Source: three-view drawing plus pictorial views. Frame: mm from the lowest corner of the part. A direction names the side the tool comes from. Give positions to 0.01 mm unless a question says otherwise; leave off trailing zeros. Loops run counter-clockwise (first coordinate to the right, second up) from the corner with the lowest first, then second, coordinate; pieces in that order, holes last.
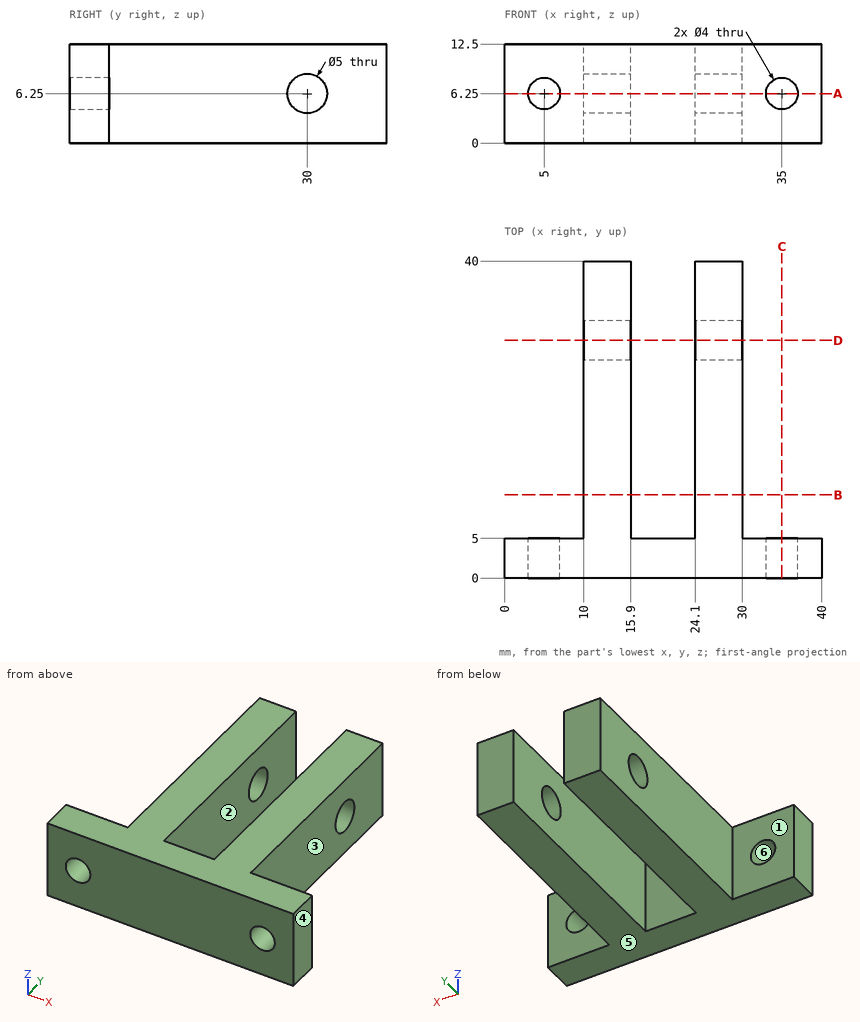
1) Ray query, probe 1 along X at (y, z) = (35.5, 4.25); probe 2 along Y at (x, z) = (9.5, 7.5); probe 3 along Y at (x, z) = (27.55, 6.25). Return the intervals inside material, ascending.
Checks:
probe 1: x = 10 to 15.9, 24.1 to 30
probe 2: y = 0 to 5
probe 3: y = 0 to 27.5, 32.5 to 40
2) Cut plane B-B (y = 10.5). Return loops of the section in (x, z).
Checks:
outline: (10, 0) - (15.9, 0) - (15.9, 12.5) - (10, 12.5) - close; (24.1, 0) - (30, 0) - (30, 12.5) - (24.1, 12.5) - close
3) Reachability of the marked faces 1, 2 and 3 from +Z, -Z, +X, -X, +Y, -Y: full face, straight path, thin tool, end or side. Return the list, or none.
Checks:
face 1: +Z, -Z, -X, +Y
face 2: +Z, -Z, +Y
face 3: +Z, -Z, +X, +Y
4) Contact query for flat-ended pins moving along their axis: P1, Ø6.5, axis at x = 5, z = 6.25, coming from the +Y side; P2, Ø1.5, axis at y = 14.5, z = 2, coming from the -X side; P3, Ø6, axis at y = 23, z = 7, coming from the +X side. Output: stop coordinate, or through.
Checks:
P1: stops at y = 5
P2: stops at x = 10
P3: stops at x = 30
5) Cut plane A-A (z = 6.25). Return loops of the section in (x, y), and give its area (3 significant figures).
Checks:
outline: (0, 0) - (3, 0) - (3, 5) - (0, 5) - close; (7, 0) - (33, 0) - (33, 5) - (30, 5) - (30, 27.5) - (24.1, 27.5) - (24.1, 5) - (15.9, 5) - (15.9, 27.5) - (10, 27.5) - (10, 5) - (7, 5) - close; (10, 32.5) - (15.9, 32.5) - (15.9, 40) - (10, 40) - close; (24.1, 32.5) - (30, 32.5) - (30, 40) - (24.1, 40) - close; (37, 0) - (40, 0) - (40, 5) - (37, 5) - close
area: 514 mm2
6) Pull-direction query (Z, two-part tool) for the marked faces 4, 5 and 6; classes: released by +Z, released by -Z, zero draft, split by the parting line, or undercut.
Checks:
face 4: zero draft
face 5: released by -Z
face 6: undercut
7) Cut plane D-D (y = 30). Return loops of the section in (x, z).
Checks:
outline: (10, 0) - (15.9, 0) - (15.9, 3.75) - (10, 3.75) - close; (10, 8.75) - (15.9, 8.75) - (15.9, 12.5) - (10, 12.5) - close; (24.1, 0) - (30, 0) - (30, 3.75) - (24.1, 3.75) - close; (24.1, 8.75) - (30, 8.75) - (30, 12.5) - (24.1, 12.5) - close
8) Cut plane C-C (x = 35). Return loops of the section in (y, z), and give its area (3 significant figures).
Checks:
outline: (0, 0) - (5, 0) - (5, 4.25) - (0, 4.25) - close; (0, 8.25) - (5, 8.25) - (5, 12.5) - (0, 12.5) - close
area: 42.5 mm2
